Work out the finished part from the listing and answer in its coordinate system (mm). Face numbers are marked on the shaded views. A direction names the side the tool comes from. Round coordinates to 2 decimals unless told otherwise and drop trailing zeros. Order: outer loops, then holes, each group sorted by start corner. A loop starts at its lowest first (then second) coordinate and runs counter-clockwise, first axis right, second up. Notation, with made-up numbers: M 12,13 L 17,13 A21 ccw 17,52 Z; hole C 35.25,0 d2. An arc over 180 degrees is marked long. Answer as a JSON object with one key per item and string values. Group by question number.
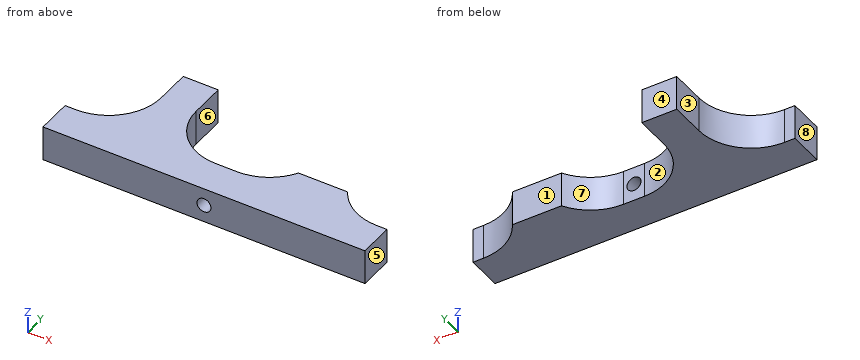
from build123d import *

# Parameters (mm, degrees)
F0_W     = 92
F0_H     = 10
F1_DEPTH = 35
F2_W     = 18
F2_H     = 25
F2_W_2   = 36
F3_DEPTH = 10
F4_R     = 2
F5_DEPTH = 10
F6_R     = 15
F7_W     = 10
F7_H     = 10
F7_W_2   = 4.897156
F7_W_3   = 5.102844
F8_DEPTH = 17.5


with BuildPart() as f1:
    # F0 (on Front) → F1 (new body)
    with BuildSketch(Plane.XZ):
        with Locations((17.840367, 26.957831)):
            Rectangle(F0_W, F0_H)
    extrude(amount=F1_DEPTH)

    # F2 (on face) → F3 (cut)
    with BuildSketch(Plane.XY.offset(31.957831)):
        with Locations((-19.159633, -12.5)):
            Rectangle(F2_W, F2_H)
        with Locations((17.840367, -12.5)):
            Rectangle(F2_W_2, F2_H)
        with Locations((54.840367, -12.5)):
            Rectangle(F2_W, F2_H)
    extrude(amount=-F3_DEPTH, mode=Mode.SUBTRACT)

    # F4 (on face) → F5 (cut)
    with BuildSketch(Plane.XZ.offset(35)):
        with Locations((17.840367, 26.957831)):
            Circle(F4_R)
    extrude(amount=-F5_DEPTH, mode=Mode.SUBTRACT)

    # F6
    f6_edges = [f1.edges().sort_by_distance(p)[0] for p in [
        (-0.159633, -25, 26.957831),
        (45.840367, -25, 26.957831),
        (35.840367, -25, 26.957831),
        (-10.159633, -25, 26.957831),
    ]]
    fillet(f6_edges, radius=F6_R)

    # F7 (on face) → F8 (cut)
    with BuildSketch(Plane(origin=(0, 0, 0), x_dir=(-1, 0, 0), z_dir=(0, 1, 0))):
        with Locations((-40.840367, 26.957831)):
            Rectangle(F7_W, F7_H)
        with Locations((-33.391789, 26.957831)):
            Rectangle(F7_W_2, F7_H)
        with Locations((-48.391789, 26.957831)):
            Rectangle(F7_W_3, F7_H)
    extrude(amount=-F8_DEPTH, mode=Mode.SUBTRACT)


solid = f1.part
Item 1: Each of these flat-tipped pins is pushed along its axis until it touches: pin 1 (5 mm diameter, centred on y = -7.5, z = 25.5, fed in from +X); pin 2 (3 mm diameter, centred on x = 17.5, z = 27, fed in from +Y); pin 3 (3.5 mm diameter, centred on x = -26, z = 28.5, fed in from +Y). Where does it stop, or does it pass through?
Item 2: Consider L1, parallel to Y at x = 35.5, z = 26.5; L2, parallel to X at y = -5.5, z = 24.25; L3, parallel to Y at x = 16, z = 25.25. Determine where each line is inside the solid, lowest interval first.
Item 3: A tool of negligible diameter and unlimited length cuts with its end or side. For the marked faces 1, 2, 3, 4 and 5, from which of +Z, -Z, +X, -X, +Y, -Y can it reach the whole face along a straight path? Write none if from no direction.
Item 4: Find section B-B (z = 23). Give the vertices of the cut face in (x, y), and give its area (3 significant figures).
Item 5: Find section A-A (y = -21). Give the vertices of the cut face in (x, z).
Item 6: Find section C-C (x = 43). Give the vertices of the cut face in (y, z).
Item 7: The mould has two halves that part along X. Classify the marked faces 6, 7 and 8: +X half, -X half, draft (parallel to the pull), parting line (faces both ways), or undercut.
Item 8: Find section D-D (y = -5.5). Give the vertices of the cut face in (x, z).
Responses:
{
 "1": {"pin 1": "stops at x = -0.16", "pin 2": "passes through", "pin 3": "stops at y = -24.97"},
 "2": {"L1": "y = -35 to -17.5", "L2": "x = -10.16 to -0.16", "L3": "y = -35 to -25"},
 "3": {"face 1": "+Z, -Z, +X, +Y", "face 2": "+Z, -Z, +Y", "face 3": "+Z, -Z, -X, +Y", "face 4": "+Z, -Z, +X, -X, +Y", "face 5": "+Z, -Z, +X, +Y, -Y"},
 "4": {"outline": "M -28.16,-35 L 63.84,-35 L 63.84,-25 L 60.84,-25 A15 cw 47.85,-17.5 L 33.83,-17.5 A15 cw 20.84,-25 L 14.84,-25 A15 cw -0.16,-10 L -0.16,0 L -10.16,0 L -10.16,-10 A15 cw -25.16,-25 L -28.16,-25 Z", "area": "1,430 mm^2"},
 "5": {"outline": "M -14.96,21.96 L 4.64,21.96 L 4.64,31.96 L -14.96,31.96 Z; M 31.04,21.96 L 50.64,21.96 L 50.64,31.96 L 31.04,31.96 Z"},
 "6": {"outline": "M -35,21.96 L -17.5,21.96 L -17.5,31.96 L -35,31.96 Z"},
 "7": {"face 6": "+X half", "face 7": "undercut", "face 8": "-X half"},
 "8": {"outline": "M -10.16,21.96 L -0.16,21.96 L -0.16,31.96 L -10.16,31.96 Z"}
}
